Work out the finished part from the listing and answer in its coordinate system (mm). Round coordinates to 2 decimals unless told otherwise and drop trailing zeros. Write each loop counter-clockwise with the first axis right and the second up, starting at its lowest first coordinate (ties: lowest second). Pieces come first, ordered by that corner, then holes. Notation, with made-up numbers: (-15, -22.5) - (29, -22.5) arc R26 ccw to (29, 2.5) - close; hole circle Ø6 at (-13.5, -16). An arc over 180 degrees is marked (long way). Write item = value, one per line. Start each with the question number.
from build123d import *

# Parameters (mm, degrees)
ESQUISSE2_W                  = 2
ESQUISSE2_H                  = 2
ESQUISSE3_R                  = 1
BOSS_EXTRU_1_DEPTH           = 2
R_P_TITION_CIRCULAIRE1_COUNT = 3


with BuildPart() as part:
    # Balayage2: sweep along a curve in space
    with BuildLine() as balayage2_path:
        Line((0, 0, 0), (0, 0, -20))
        Line((0, 0, -20), (0, 60, -20))
    # Esquisse2 → Balayage2 (sweep)
    with BuildSketch(Plane.XY):
        Rectangle(ESQUISSE2_W, ESQUISSE2_H)
    balayage2 = sweep(path=balayage2_path.line, transition=Transition.RIGHT)

    # Esquisse3 → Boss.-Extru.1 (add, symmetric)
    with BuildSketch(Plane(origin=(0, 0, 0), x_dir=(1, 0, 0), z_dir=(0, 1, 0))):
        with Locations(Location((0, 0, 0), (0, 0, 270))):
            Circle(ESQUISSE3_R)
    extrude(amount=BOSS_EXTRU_1_DEPTH, both=True)

    # Répétition circulaire1: Balayage2 ×3 about axis
    r_p_tition_circulaire1_axis = Axis((0, 0, 0), (0, 1, 0))
    for i in range(1, R_P_TITION_CIRCULAIRE1_COUNT):
        add(balayage2.rotate(r_p_tition_circulaire1_axis, i * 360 / R_P_TITION_CIRCULAIRE1_COUNT))


solid = part.part
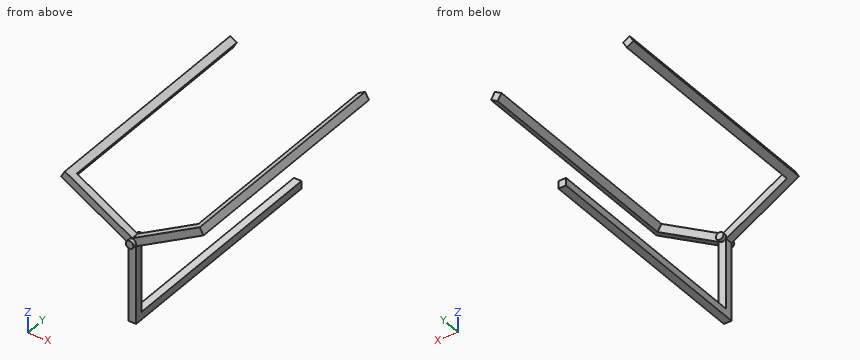
1. Find section A-A on y = 45.5. Give the vertices of the cut face in (x, z).
2. Each of these flat-tipped pins is pushed along its axis until it touches: pin 1 (1.6 mm diameter, centred on x = 0, y = 26, fed in from +Z); pin 2 (1.6 mm diameter, centred on x = -0.5, z = 0, fed in from +Y); pin 3 (1 mm diameter, centred on x = -14.5, y = 20, fed in from -Z); pin 4 (10 mm diameter, centred on y = 15, z = -15, fed in from -X). Where does it stop, or does it pass through?
3. Find section C-C on x = -11. Give the vertices of the cut face in (y, z).
4. Consider line 1 (X direction, y = 22, z = 9); line 2 (Y direction, x = -0.5, z = -2); line 3 (Z direction, x = -17, y = 37.5). Determine where each line is inside the solid, lowest interval first.
5. Find section B-B on z = -12.5. Give the vertices of the cut face in (x, y), plus the area to 3 significant figures.
Answer key:
q1.outline = (-18.69, 9.63) - (-16.95, 8.63) - (-15.95, 10.37) - (-17.69, 11.37) - close; (-1, -21) - (1, -21) - (1, -19) - (-1, -19) - close; (15.95, 10.37) - (16.95, 8.63) - (18.69, 9.63) - (17.69, 11.37) - close
q2.pin_1 = -19
q2.pin_2 = 2
q2.pin_3 = through
q2.pin_4 = -1
q3.outline = (-1, 5.2) - (1, 5.2) - (1, 7.51) - (-1, 7.51) - close
q4.line_1 = -17.59 to -16.74, 16.74 to 17.59
q4.line_2 = -1 to 1
q4.line_3 = 8.66 to 10.97
q5.outline = (-1, -1) - (1, -1) - (1, 1) - (-1, 1) - close
q5.area = 4.00 mm²
